```python
from build123d import *

# Parameters (mm, degrees)
FILLET1_R      = 2
CHAMFER2_SIZE  = 1.5
CHAMFER2_SIZE2 = 0.866025404


with BuildPart() as part:
    # Sketch4 → Revolve1 (revolve)
    with BuildSketch(Plane.XY, mode=Mode.PRIVATE) as revolve1_sk:
        Polygon((0, 0), (3.95, 0), (3.95, 10), (2.95, 10), (2.95, 36.5), (0, 36.5), align=None)
    revolve(revolve1_sk.sketch.rotate(Axis((0, 0, 0), (0, 1, 0)), 90), axis=Axis((0, 0, 0), (0, 1, 0)))

    # Fillet1
    fillet1_edges = [part.edges().sort_by_distance(p)[0] for p in [
        (0, 36.5, 2.95),
    ]]
    fillet(fillet1_edges, radius=FILLET1_R)

    # Chamfer2
    chamfer2_edges = [part.edges().sort_by_distance(p)[0] for p in [
        (0, 0, 3.95),
    ]]
    chamfer2_side = [part.faces().sort_by_distance(p)[0] for p in [
        (0, 5, 3.95),
    ]]
    chamfer(chamfer2_edges, length=CHAMFER2_SIZE, length2=CHAMFER2_SIZE2, reference=chamfer2_side[0])


solid = part.part
```
Source: CAD feature listing. Evaluate the final solid. Frame: model axes, mm. A direction names the side the tool comes from. Round coordinates to 2 decimals unless told otherwise and drop trailing zeros. Order: outer loops, then holes, each group sorted by start corner. A loop starts at its lowest first (then second) coordinate and runs counter-clockwise, first axis right, second up. Notation, with made-up numbers: (17.5, -9.75) -> (25.5, -9.75) arc R27 ccw to (25.5, 25.25) -> close; hole circle Ø4 at (10.5, 72.5). An arc over 180 degrees is marked (long way). One line per item, written item: value. Start each with the question number.
Q1. Access query for faces 1 (the flat face through (3, 10, 1)), 2 (the flat face through (0, 0, 0)). Directions: +Z, -Z, +X, -X, +Y, -Y. A direction counts if a zero-diameter tool reaches every point of the face in a straight line with its end or side. Return the directions, or none.
Q2. Pin query (flat end, axial travel): pin 1 (1.5 mm diameter, centred on y = 7.5, z = 2.5, fed in from +X). Return the tip coordinate at first contact, or that it passes through.
Q3. Section query B-B (y = 25). Return the cut outline in (x, z).
Q4. Material intervals for probe 1 along Z at (x, y) = (0.25, 5); probe 2 along Y at (x, z) = (-1, 0.25); probe 3 along Z at (x, y) = (1, 24), sorted ascending.
Q5. Section query A-A (y = 6.5). Return the cut outline in (x, z), plus the area to 3 significant figures.
Findings below:
1. face 1: +Y
1. face 2: +Z, -Z, +X, -X, -Y
2. pin 1: x = 3.54
3. outline: circle Ø5.9 at (0, 0)
4. probe 1: -3.94 to 3.94
4. probe 2: 0 to 36.5
4. probe 3: -2.78 to 2.78
5. outline: circle Ø7.9 at (0, 0)
5. area: 49.0 mm²
